Check sheet for the modelled part. Datum: model origin and axes. Units: mm. A direction names the side the tool comes from. Coordinates: 2 decimals unless noted, no trailing zeros. Loops run counter-clockwise (first coordinate to the right, second up) from the corner with the lowest first, then second, coordinate; pieces in that order, holes last. Notation, with made-up numbers: (84, 72.25) -> (103, 72.25) arc R7 cw to (103, 76.25) -> close; hole circle Ø11 at (8, 43.25). An arc over 180 degrees is marked (long way). Use CSV: the item, a comma, the result in double quotes. Start each with the question number.
1. Sectioned sample at A-A, the plane z = 15. Record the cut outline in (x, y), and give its area (3 significant figures).
2. Set-up check for faces 5 (the face through (0, 12, 0)), 6 (the face through (-10, 0, -20)), 7 (the face through (0, -6, 23)), 8 (the face through (0, -10, -20)): record each of +Z, -Z, +X, -X, +Y, -Y from which the full face is reachable in a straight line by a thin tool's end or side.
3. Sectioned sample at C-C, the plane x = -3. Record the cut outline in (y, z).
4. Gauge pin test, flat ends, axial feed: pin 1 (4 mm diameter, centred on x = 1.5, z = -47, fed in from -Y); pin 2 (8 mm diameter, centred on y = 6, z = -35.5, fed in from +X); pin 3 (0.7 mm diameter, centred on x = 19.5, y = 4.5, fed in from -Z). Record the tip position at first contact, or that the pin passes through.
5. Sectioned sample at B-B, the plane y = 1.5. Record the cut outline in (x, z), and give its area (3 significant figures).
6. Release check for a two-part mould opening along Z. For faces 1 (the face through (16.056, 0.084, 23.171)), 2 (the face through (-2.17, -9.76, -52.18)), 3 (the face through (-1.301, 0.084, 52.857)), 4 (the face through (-8, -8, -30)) record: pulls with the +Z half, pulls with the -Z half, needs draft (parallel to the pull), parting line crosses it, or undercut.
7. Thickness scan on L1, parallel to Z at x = 0, y = -1; L2, parallel to Y at x = -8, z = 27; L3, parallel to Z at x = 13, y = -9.5. Record the ranges inside material, lowest first.
8. Sectioned sample at D-D, the plane z = -18. Record the cut outline in (x, y), and give its area (3 significant figures).
Solid Edge part; units mm, degrees
sketch "Sketch1" plane through (0, 0, 0) normal (0, -1, 0) x (1, 0, 0)
  circle A0 centre (0, 47) radius 6
  line L0 (-20, 0) -> (20, 0)
  line L1 (20, 0) -> (12, 47)
  line L2 (-20, 0) -> (-12, 47)
  arc A1 (12, 47) -> (-12, 47) centre (0, 47) ccw
  circle A2 centre (0, 15) radius 6
  dimension "D1" = 20
extrude "Protrusion1" add sketch "Sketch1" along normal mid plane 12
sketch "Sketch2" plane through (0, 0, 0) normal (0, 0, 1) x (1, 0, 0)
  circle A0 centre (0, 0) radius 20
extrude "ExtrudedProtrusion_6" add sketch "Sketch2" against normal blind 10
sketch "Sketch3" plane through (0, 0, -10) normal (0, 0, -1) x (1, 0, 0)
  line L0 (-10, 10) -> (10, 10)
  line L1 (10, 10) -> (10, -10)
  line L2 (10, -10) -> (-10, -10)
  line L3 (-10, -10) -> (-10, 10)
  dimension "D1" = 10
  dimension "D2" = 10
extrude "ExtrudedProtrusion_7" add sketch "Sketch3" along normal blind 20
sketch "Sketch4" plane through (0, 0, -30) normal (0, 0, -1) x (1, 0, 0)
  circle A0 centre (0, 0) radius 10
extrude "ExtrudedProtrusion_8" add sketch "Sketch4" along normal blind 45
cosmetic_thread "Thread1"
properties part number "3" material "Fe 410 W"
Completed:
1,outline,"(-17.45, -6) -> (-6, -6) -> (-6, 6) -> (-17.45, 6) -> close; (6, -6) -> (17.45, -6) -> (17.45, 6) -> (6, 6) -> close"
1,area,"275 mm²"
2,face 5,"+Z, +X, -X, +Y"
2,face 6,"-Z, -X, +Y, -Y"
2,face 7,"+Z, +X, -X, -Y"
2,face 8,"-Z, +X, -X, -Y"
3,outline,"(-19.77, -10) -> (-10, -10) -> (-10, -30) -> (-9.54, -30) -> (-9.54, -75) -> (9.54, -75) -> (9.54, -30) -> (10, -30) -> (10, -10) -> (19.77, -10) -> (19.77, 0) -> (6, 0) -> (6, 9.8) -> (-6, 9.8) -> (-6, 0) -> (-19.77, 0) -> close; (-6, 20.2) -> (6, 20.2) -> (6, 41.8) -> (-6, 41.8) -> close; (-6, 52.2) -> (6, 52.2) -> (6, 58.62) -> (-6, 58.62) -> close"
4,pin 1,"y = -10"
4,pin 2,"x = 9.8"
4,pin 3,"z = -10"
5,outline,"(-20, 0) -> (-19.94, 0) -> (-19.94, -10) -> (-10, -10) -> (-10, -30) -> (-9.89, -30) -> (-9.89, -75) -> (9.89, -75) -> (9.89, -30) -> (10, -30) -> (10, -10) -> (19.94, -10) -> (19.94, 0) -> (20, 0) -> (12, 47) arc R12 ccw to (-12, 47) -> close; hole circle Ø12 at (0, 15); hole circle Ø12 at (0, 47)"
5,area,"3,190 mm²"
6,face 1,"pulls with the +Z half"
6,face 2,"needs draft"
6,face 3,"undercut"
6,face 4,"pulls with the -Z half"
7,L1,"-75 to 9, 21 to 41, 53 to 59"
7,L2,"-6 to 6"
7,L3,"-10 to 0"
8,outline,"(-10, -10) -> (10, -10) -> (10, 10) -> (-10, 10) -> close"
8,area,"400 mm²"
